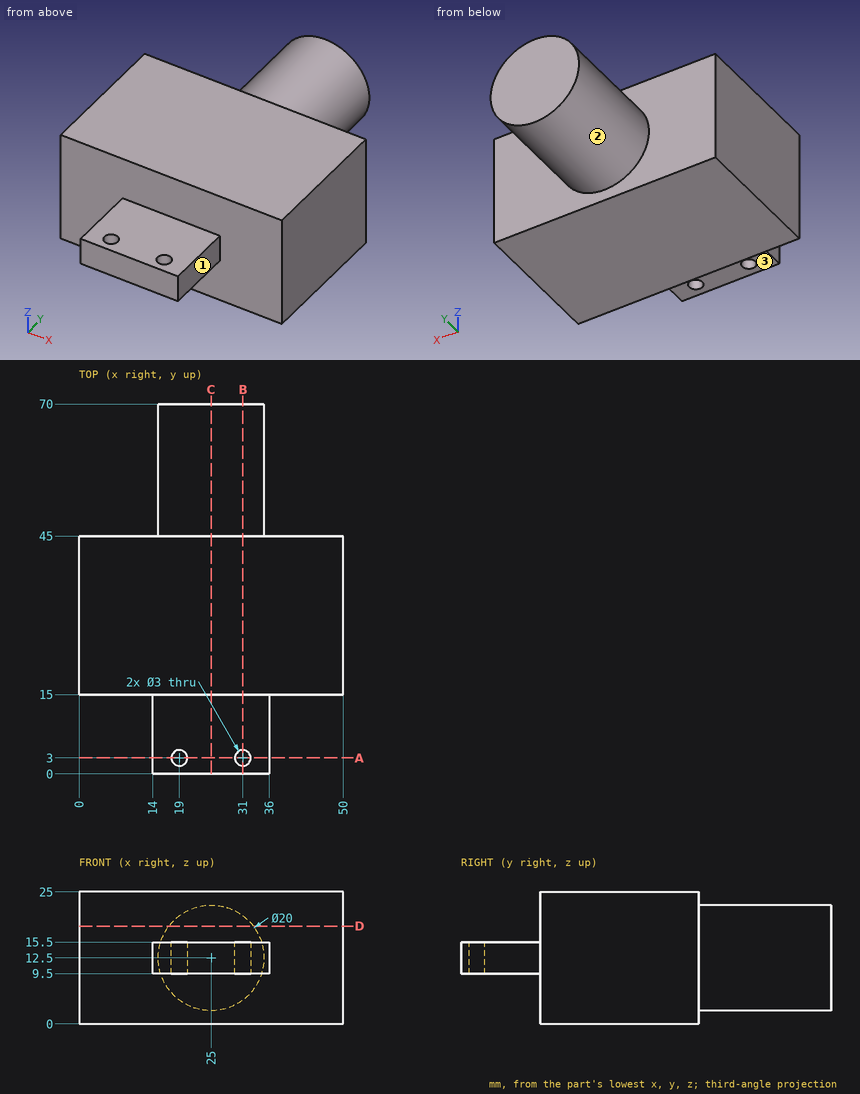
Study the drawing (mm; zero at the part's minimum x, y, z) and answer. A direction names the side the tool comes from. Round coordinates to 2 decimals unless told otherwise and drop trailing zeros. Order: outer loops, then holes, each group sorted by start corner. A loop starts at its lowest first (then second) coordinate and runs counter-clockwise, first axis right, second up. Notation, with made-up numbers: M 87.5,20.5 L 92.5,20.5 A14 ccw 92.5,24.5 Z; hole C -36.75,74.25 d10. An arc over 180 degrees is marked long. One line per item, written item: value.
Q1. Flat-ended cylindrical pins translate along their axes: pin 1 (5 mm diameter, centred on x = 31, y = 3, fed in from -Z); pin 2 (16.5 mm diameter, centred on x = 29, y = 4.5, fed in from +Z); pin 3 (6.5 mm diameter, centred on y = 5.5, z = 14, fed in from -X); pin 4 (10 mm diameter, centred on y = 9.5, z = 3, fed in from +X). Find the tip coordinate at first contact, or state that the pin passes through.
Derived:
pin 1: z = 9.5
pin 2: z = 15.5
pin 3: x = 14
pin 4: through
Q2. Find section B-B on x = 31. Write down the section's boundary in (y, z).
Derived:
outline: M 0,9.5 L 1.5,9.5 L 1.5,15.5 L 0,15.5 Z; M 4.5,9.5 L 15,9.5 L 15,0 L 45,0 L 45,4.5 L 70,4.5 L 70,20.5 L 45,20.5 L 45,25 L 15,25 L 15,15.5 L 4.5,15.5 Z
Q3. Find section A-A on y = 3. Write down the section's boundary in (x, z).
Derived:
outline: M 14,9.5 L 17.5,9.5 L 17.5,15.5 L 14,15.5 Z; M 20.5,9.5 L 29.5,9.5 L 29.5,15.5 L 20.5,15.5 Z; M 32.5,9.5 L 36,9.5 L 36,15.5 L 32.5,15.5 Z
Q4. Straight lines are drawn through the part: line 1 (Y direction, x = 31, z = 14); line 2 (Y direction, x = 24, z = 23); line 3 (Y direction, x = 19, z = 17.5). For each, find the intervals that lie inside material, in ascending order.
Derived:
line 1: 0 to 1.5, 4.5 to 70
line 2: 15 to 45
line 3: 15 to 70
Q5. Find section C-C on x = 25. Write down the section's boundary in (y, z).
Derived:
outline: M 0,9.5 L 15,9.5 L 15,0 L 45,0 L 45,2.5 L 70,2.5 L 70,22.5 L 45,22.5 L 45,25 L 15,25 L 15,15.5 L 0,15.5 Z
Q6. For the marked faces 1, 2 and 3, determine the directions among +Z, -Z, +X, -X, +Y, -Y from which every point of the face is accessible in a straight line to the end or side of a thin tool.
Derived:
face 1: +Z, -Z, +X, -Y
face 2: +Y
face 3: -Z, +X, -X, -Y
Q7. Find section D-D on z = 18.5. Write down the section's boundary in (x, y), then the cut area to 3 significant figures.
Derived:
outline: M 0,15 L 50,15 L 50,45 L 33,45 L 33,70 L 17,70 L 17,45 L 0,45 Z
area: 1,900 mm²
